The model under review builds one solid part; all positions refer to its coordinate system, in mm. Coordinates: 2 decimals unless noted, no trailing zeros. Order: outer loops, then holes, each group sorted by start corner. A loop starts at its lowest first (then second) coordinate and runs counter-clockwise, first axis right, second up.
```python
from build123d import *

# Parameters (mm, degrees)
CROQUIS1_W              = 99
CROQUIS1_H              = 99
CROQUIS1_W_2            = 96
CROQUIS1_H_2            = 96
SALIENTE_EXTRUIR1_DEPTH = 2
CROQUIS2_W              = 96
CROQUIS2_H              = 5
CROQUIS2_H_2            = 8.6
SALIENTE_EXTRUIR2_DEPTH = 1
CROQUIS3_W              = 105
CROQUIS3_H              = 105
CROQUIS3_W_2            = 99
CROQUIS3_H_2            = 99
SALIENTE_EXTRUIR3_DEPTH = 1
CROQUIS6_W              = 96
CROQUIS6_H              = 96
SALIENTE_EXTRUIR5_DEPTH = 1
CROQUIS7_W              = 60.769249784
CROQUIS7_H              = 60.769249784
CROQUIS7_W_2            = 57.769249784
CROQUIS7_H_2            = 57.769249784
SALIENTE_EXTRUIR6_DEPTH = 2
CROQUIS8_W              = 10
CROQUIS8_H              = 7
CROQUIS8_W_2            = 7
CROQUIS8_H_2            = 10
CORTAR_EXTRUIR1_DEPTH   = 65
CROQUIS9_W              = 99
CROQUIS9_H              = 99
CROQUIS9_W_2            = 96
CROQUIS9_H_2            = 96
SALIENTE_EXTRUIR7_DEPTH = 1


with BuildPart() as part:
    # Croquis1 → Saliente-Extruir1 (new body)
    with BuildSketch(Plane(origin=(0, 0, 0), x_dir=(1, 0, 0), z_dir=(0, 1, 0))):
        with Locations((49.5, 49.5)):
            Rectangle(CROQUIS1_W, CROQUIS1_H)
        with Locations((49.5, 49.5)):
            Rectangle(CROQUIS1_W_2, CROQUIS1_H_2, mode=Mode.SUBTRACT)
    extrude(amount=SALIENTE_EXTRUIR1_DEPTH)

    # Croquis2 → Saliente-Extruir2 (add)
    with BuildSketch(Plane.XZ):
        with Locations((49.5, -52)):
            Rectangle(CROQUIS2_W, CROQUIS2_H)
        with Locations((49.5, -47)):
            Rectangle(CROQUIS2_W, CROQUIS2_H)
        with Locations((49.5, -67.4)):
            Rectangle(CROQUIS2_W, CROQUIS2_H_2)
        with Locations((49.5, -84.6)):
            Rectangle(CROQUIS2_W, CROQUIS2_H_2)
        with Locations((49.5, -31.6)):
            Rectangle(CROQUIS2_W, CROQUIS2_H_2)
        with Locations((49.5, -14.4)):
            Rectangle(CROQUIS2_W, CROQUIS2_H_2)
    extrude(amount=-SALIENTE_EXTRUIR2_DEPTH)

    # Croquis3 → Saliente-Extruir3 (add)
    with BuildSketch(Plane.XZ):
        with Locations((49.5, -49.5)):
            Rectangle(CROQUIS3_W, CROQUIS3_H)
        with Locations((49.5, -49.5)):
            Rectangle(CROQUIS3_W_2, CROQUIS3_H_2, mode=Mode.SUBTRACT)
    extrude(amount=-SALIENTE_EXTRUIR3_DEPTH)

    # Croquis6 → Saliente-Extruir5 (add)
    with BuildSketch(Plane(origin=(0, 1, 0), x_dir=(1, 0, 0), z_dir=(0, 1, 0))):
        with Locations((49.5, 49.5)):
            Rectangle(CROQUIS6_W, CROQUIS6_H)
    extrude(amount=-SALIENTE_EXTRUIR5_DEPTH)

    # Croquis7 → Saliente-Extruir6 (add)
    with BuildSketch(Plane(origin=(0, 1, 0), x_dir=(1, 0, 0), z_dir=(0, 1, 0))):
        with Locations((49.5, 49.5)):
            Rectangle(CROQUIS7_W, CROQUIS7_H)
        with Locations((49.5, 49.5)):
            Rectangle(CROQUIS7_W_2, CROQUIS7_H_2, mode=Mode.SUBTRACT)
    extrude(amount=SALIENTE_EXTRUIR6_DEPTH)

    # Croquis8 → Cortar-Extruir1 (cut)
    with BuildSketch(Plane(origin=(0, 1, 0), x_dir=(1, 0, 0), z_dir=(0, 1, 0))):
        with Locations((49.5, 11.615375108)):
            Rectangle(CROQUIS8_W, CROQUIS8_H)
        with Locations((11.615375108, 49.5)):
            Rectangle(CROQUIS8_W_2, CROQUIS8_H_2)
        with Locations((49.5, 87.384624892)):
            Rectangle(CROQUIS8_W, CROQUIS8_H)
        with Locations((87.384624892, 49.5)):
            Rectangle(CROQUIS8_W_2, CROQUIS8_H_2)
    extrude(amount=-CORTAR_EXTRUIR1_DEPTH, mode=Mode.SUBTRACT)

    # Croquis9 → Saliente-Extruir7 (add)
    with BuildSketch(Plane(origin=(0, 2, 0), x_dir=(1, 0, 0), z_dir=(0, 1, 0))):
        with Locations((49.5, 49.5)):
            Rectangle(CROQUIS9_W, CROQUIS9_H)
        with Locations((49.5, 49.5)):
            Rectangle(CROQUIS9_W_2, CROQUIS9_H_2, mode=Mode.SUBTRACT)
    extrude(amount=SALIENTE_EXTRUIR7_DEPTH)


solid = part.part
```
(1) We need section B-B, the plane x = 48. Write out the cut boundary in (y, z).
A:
outline: (0, -102) - (1, -102) - (1, -99) - (3, -99) - (3, -97.5) - (1, -97.5) - (1, -90.88) - (0, -90.88) - close; (0, -83.88) - (1, -83.88) - (1, -79.88) - (3, -79.88) - (3, -78.38) - (1, -78.38) - (1, -20.62) - (3, -20.62) - (3, -19.12) - (1, -19.12) - (1, -15.12) - (0, -15.12) - close; (0, -8.12) - (1, -8.12) - (1, -1.5) - (3, -1.5) - (3, 0) - (1, 0) - (1, 3) - (0, 3) - close
(2) We need section C-C, the plane x = 87. Write out the cut boundary in (y, z), and give its area (3 significant figures).
A:
outline: (0, -102) - (1, -102) - (1, -99) - (3, -99) - (3, -97.5) - (1, -97.5) - (1, -54.5) - (0, -54.5) - close; (0, -44.5) - (1, -44.5) - (1, -1.5) - (3, -1.5) - (3, 0) - (1, 0) - (1, 3) - (0, 3) - close
area: 101 mm2
(3) Wall thickness on probe 1 along Z at (x, y) = (52, 0.65); probe 2 along X at (y, z) = (1.9, -28.5); probe 3 along Z at (x, y) = (71.5, 2.2): over which ranges is each line inside the solid? List them lowest first.
A:
probe 1: z = -102 to -90.88, -83.88 to -15.12, -8.12 to 3
probe 2: x = 0 to 1.5, 19.12 to 20.62, 78.38 to 79.88, 97.5 to 99
probe 3: z = -99 to -97.5, -79.88 to -78.38, -20.62 to -19.12, -1.5 to 0
(4) For pin 1 Ø4 at (x, z) = (24, -38) entering from +Y; pin 2 Ø0.6 at (y, z) = (1.5, -41) entering from +X; pin 3 Ø1.6 at (y, z) = (2.5, -53.5) entering from -X, all flat-tipped, find the tip position at first contact; note any pin that passes through.
A:
pin 1: stops at y = 1
pin 2: stops at x = 99
pin 3: stops at x = 0
(5) Draft analysis for pull direction Z (two halves, no side actions). For faces 1 (the face through (49, 1, -50)), 2 (the face through (49, 0, -50)), state which applies: released by +Z, released by -Z, zero draft, split by the parting line, or undercut.
A:
face 1: undercut
face 2: zero draft
(6) We need section D-D, the plane z = -24. Write out the cut boundary in (x, y).
A:
outline: (-3, 0) - (102, 0) - (102, 1) - (99, 1) - (99, 3) - (97.5, 3) - (97.5, 1) - (79.88, 1) - (79.88, 3) - (78.38, 3) - (78.38, 1) - (20.62, 1) - (20.62, 3) - (19.12, 3) - (19.12, 1) - (1.5, 1) - (1.5, 3) - (0, 3) - (0, 1) - (-3, 1) - close
(7) We need section A-A, the plane y = 1.9. Write out the cut boundary in (x, z), and give its area (3 significant figures).
A:
outline: (0, -99) - (99, -99) - (99, 0) - (0, 0) - close; (19.12, -79.88) - (79.88, -79.88) - (79.88, -19.12) - (19.12, -19.12) - close; hole (1.5, -97.5) - (97.5, -97.5) - (97.5, -1.5) - (1.5, -1.5) - close; hole (20.62, -78.38) - (78.38, -78.38) - (78.38, -20.62) - (20.62, -20.62) - close
area: 941 mm2
